Autodesk Inventor part; units mm, degrees
ref_plane "YZ Plane" through (0, 0, 0) normal (1, 0, 0) x (0, 1, 0)
ref_plane "XZ Plane" through (0, 0, 0) normal (0, 1, 0) x (-1, 0, 0)
ref_plane "XY Plane" through (0, 0, 0) normal (0, 0, 1) x (1, 0, 0)
sketch "Esquisse2" plane through (0, 0, 0) normal (0, 0, 1) x (1, 0, 0)
  line L0 (0, 17.0922) -> (0, -5.3775) construction
  line L1 (0, 0) -> (7.5, 0)
  line L2 (7.5, 0) -> (7.5, 1)
  line L3 (7.5, 1) -> (5.5, 1)
  line L4 (5.5, 1) -> (5.5, 13)
  line L5 (5.5, 13) -> (7.5, 13)
  line L6 (7.5, 13) -> (7.5, 14)
  line L7 (7.5, 14) -> (0, 14)
  line L8 (0, 14) -> (0, 0)
  dimension "d8" = 15
  dimension "d9" = 1
  dimension "d10" = 1
  dimension "d11" = 14
  dimension "d12" = 2
  dimension "d20" = 7.5
revolve "Révolution1" add sketch "Esquisse2" angle 360 about axis through (0, 17.0922, 0) along (0, -1, 0)
sketch "Esquisse3" plane through (0, 14, 0) normal (0, 1, 0) x (1, 0, 0)
  point P0 (0, 0)
  point P1 (0, 0)
hole "Perçage1" at (0, 14, 0) direction (0, -1, 0) diameter 3.1 end through all
equation "\"d20\" = 0.5 * d8"
properties part number "poulie courroie"
Build history of the part. All positions in model axes, mm. A direction names the side the tool comes from. Round coordinates to 2 decimals unless told otherwise and drop trailing zeros. Write each loop counter-clockwise with the first axis right and the second up, starting at its lowest first coordinate (ties: lowest second). Pieces come first, ordered by that corner, then holes. Notation, with made-up numbers: (12.5, 67) - (54.5, 67) arc R13 ccw to (54.5, 71) - close; hole circle Ø5 at (33, 24). An arc over 180 degrees is marked (long way). Answer as CSV lines item,"result".
Q1. Cut at B-B (z = 0). Write the cut outline in (x, y), and give its area (3 significant figures).
Report:
outline,"(-7.5, 0) - (-1.55, 0) - (-1.55, 14) - (-7.5, 14) - (-7.5, 13) - (-5.5, 13) - (-5.5, 1) - (-7.5, 1) - close; (1.55, 0) - (7.5, 0) - (7.5, 1) - (5.5, 1) - (5.5, 13) - (7.5, 13) - (7.5, 14) - (1.55, 14) - close"
area,"119 mm^2"
Q2. Cut at C-C (y = 11.5). Write the cut outline in (x, z), and give its area (3 significant figures).
Report:
outline,"circle Ø11 at (0, 0); hole circle Ø3.1 at (0, 0)"
area,"87.5 mm^2"
Q3. Cut at A-A (x = 0). Write the cut outline in (y, z), and give its area (3 significant figures).
Report:
outline,"(0, -7.5) - (1, -7.5) - (1, -5.5) - (13, -5.5) - (13, -7.5) - (14, -7.5) - (14, -1.55) - (0, -1.55) - close; (0, 1.55) - (14, 1.55) - (14, 7.5) - (13, 7.5) - (13, 5.5) - (1, 5.5) - (1, 7.5) - (0, 7.5) - close"
area,"119 mm^2"
Q4. Drill centre lines: probe 1 along Z at (x, y) = (0, 8); probe 2 along Y at (x, z) = (-5.5, 2.25); probe 3 along Z at (x, y) = (3.25, 12.75). Where is each one in solid material? Low to high. Write a range as [from, to].
Report:
probe 1,"z = [-5.5, -1.55], [1.55, 5.5]"
probe 2,"y = [0, 1], [13, 14]"
probe 3,"z = [-4.44, 4.44]"
Q5. Pull direction Y, two halves, no side cores. Call faces 1 (the cylindrical face through (-1.19, 7.08, 5.37)), 2 (the flat face through (0, 0, -2)), 3 (the cylindrical face through (1.375, 6.902, 0.715)): +Y half, -Y half, draft (parallel to the pull), parting line (faces both ways), or undercut.
Report:
face 1,"undercut"
face 2,"-Y half"
face 3,"draft"
Q6. Cut at D-D (x = 6). Write the cut outline in (y, z), and give its area (3 significant figures).
Report:
outline,"(0, -4.5) - (1, -4.5) - (1, 4.5) - (0, 4.5) - close; (13, -4.5) - (14, -4.5) - (14, 4.5) - (13, 4.5) - close"
area,"18.0 mm^2"
Q7. Drop flat-ended pins along their axis: pin 1 (1.5 mm diameter, centred on x = 3, y = 6.5, fed in from +Z); pin 2 (1.5 mm diameter, centred on y = 5.5, z = -5.5, fed in from +X); pin 3 (1 mm diameter, centred on x = 1, y = 3.5, fed in from -Z). Give the stop position or say it passes through.
Report:
pin 1,"stops at z = 5.02"
pin 2,"stops at x = 2.77"
pin 3,"stops at z = -5.48"
Q8. Tool access for faces 4 (the flat face through (-4, 13, 4)), 5 (the cylindrical face through (-7.493, 13.507, -0.33)): list every direction of +Z, -Z, +X, -X, +Y, -Y with a clear straight run to the whole face (end or side of a thin tool).
Report:
face 4,"none"
face 5,"+Y, -Y"
